```python
from build123d import *

# Parameters (mm, degrees)
F0_W     = 57.15
F0_H     = 44.45
F1_DEPTH = 25.4
F3_DEPTH = 25.401
F5_DEPTH = 12.7


with BuildPart() as f1:
    # F0 (on Front) → F1 (new body)
    with BuildSketch(Plane.XZ):
        with Locations((28.575, 22.225)):
            Rectangle(F0_W, F0_H)
    extrude(amount=F1_DEPTH)

    # F2 (on face) → F3 (cut, through all)
    with BuildSketch(Plane.XZ.offset(25.4)):
        with BuildLine():
            ThreePointArc((35.892886882, 31.75), (31.1184848556, 40.0408067571), (21.5512819933, 40.0727565117))
            Line((21.5512819933, 40.0727565117), (26.3071428571, 31.75))
            Line((26.3071428571, 31.75), (35.892886882, 31.75))
        make_face()
        with BuildLine():
            Line((26.3071428571, 31.75), (21.5512819933, 40.0727565117))
            ThreePointArc((21.5512819933, 40.0727565117), (18.0163361, 36.5613419984), (16.7213988323, 31.75))
            Line((16.7213988323, 31.75), (26.3071428571, 31.75))
        make_face()
        with BuildLine():
            Line((31.063003721, 23.4272434883), (26.3071428571, 31.75))
            Line((26.3071428571, 31.75), (16.7213988323, 31.75))
            ThreePointArc((16.7213988323, 31.75), (21.4958008587, 23.4591932429), (31.063003721, 23.4272434883))
        make_face()
        with BuildLine():
            Line((35.892886882, 31.75), (26.3071428571, 31.75))
            Line((26.3071428571, 31.75), (31.063003721, 23.4272434883))
            ThreePointArc((31.063003721, 23.4272434883), (34.5979496143, 26.9386580016), (35.892886882, 31.75))
        make_face()
    extrude(amount=-F3_DEPTH, mode=Mode.SUBTRACT)

    # F4 (on face) → F5 (cut)
    with BuildSketch(Plane.XZ.offset(25.4)):
        with BuildLine():
            Line((57.15, 44.45), (19.05, 44.45))
            Line((19.05, 44.45), (21.5512819933, 40.0727565117))
            ThreePointArc((21.5512819933, 40.0727565117), (31.1184848556, 40.0408067571), (35.892886882, 31.75))
            ThreePointArc((35.892886882, 31.75), (34.5979496143, 26.9386580016), (31.063003721, 23.4272434883))
            Line((31.063003721, 23.4272434883), (44.45, 0))
            Line((44.45, 0), (57.15, 0))
            Line((57.15, 0), (57.15, 44.45))
        make_face()
    extrude(amount=-F5_DEPTH, mode=Mode.SUBTRACT)


solid = f1.part
```
Here's how the part is built. I have some questions about the finished solid (model axes, mm). A direction names the side the tool comes from. Coordinates: 2 decimals unless noted, no trailing zeros. Order: outer loops, then holes, each group sorted by start corner. A loop starts at its lowest first (then second) coordinate and runs counter-clockwise, first axis right, second up.
1) Imagine slicing it at C-C on z = 37.5. List the corners of the cut face in (x, y) for me.
2) Will this pin go through, and if not, where does the flat tip stop? pin 1 (3 mm diameter, centred on y = -19, z = 11, fed in from +X).
3) I need wall thicknesses on line 1 (X direction, y = -5.25, z = 31.5); line 2 (Y direction, x = 37, z = 23.5); line 3 (X direction, y = -7.25, z = 37). Which ranges of each line are inside material? Lowest first, please.
4) Which directions (+Z, -Z, +X, -X, +Y, -Y) give clear straight access to the entire face, cutting with the end or side of a thin tool? Please do faces 1 (the face through (20.283, -19.139, 42.292)), 2 (the face through (28, 0, 18)).
5) Imagine slicing it at A-A on x = 34.5. List the corners of the cut face in (y, z) for me.
6) Imagine slicing it at D-D on y = -3.5. List the corners of the cut face in (x, z) for me.
Response values:
1. outline: (0, -25.4) - (18.64, -25.4) - (18.64, 0) - (0, 0) - close; (33.98, -12.7) - (57.15, -12.7) - (57.15, 0) - (33.98, 0) - close
2. pin 1: stops at x = 39.02
3. line 1: x = 0 to 16.72, 35.89 to 57.15
3. line 2: y = -12.7 to 0
3. line 3: x = 0 to 18.29, 34.33 to 57.15
4. face 1: +Z, +X, -Y
4. face 2: +Z, -Z, +X, -X, +Y
5. outline: (-25.4, 0) - (0, 0) - (0, 26.77) - (-12.7, 26.77) - (-12.7, 17.41) - (-25.4, 17.41) - close; (-12.7, 36.73) - (0, 36.73) - (0, 44.45) - (-12.7, 44.45) - close
6. outline: (0, 0) - (57.15, 0) - (57.15, 44.45) - (0, 44.45) - close; hole circle Ø19.17 at (26.31, 31.75)
